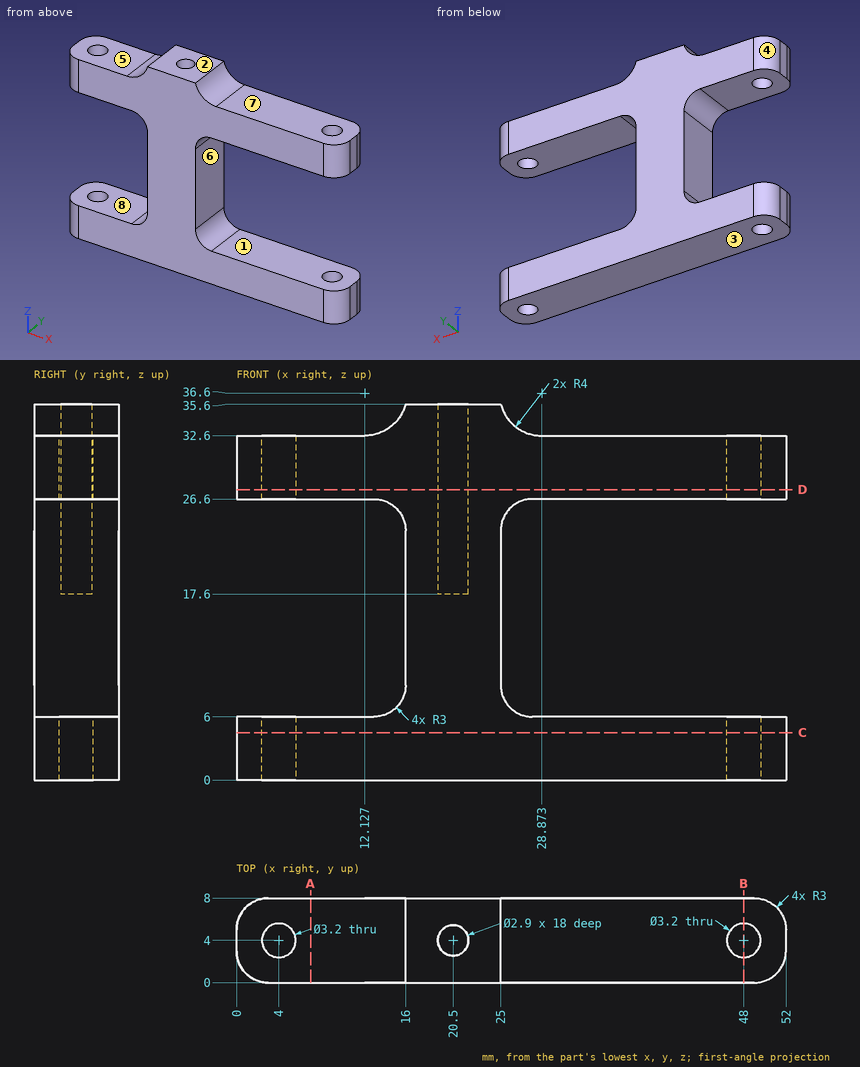
Study the drawing (mm; zero at the part's minimum x, y, z) and answer. A direction names the side the tool comes from. Round coordinates to 2 decimals unless told otherwise and drop trailing zeros. Write each loop counter-clockwise with the first axis right and the second up, starting at its lowest first coordinate (ties: lowest second). Pieces come first, ordered by that corner, then holes.
Q1. The mould has two halves that part along Z. Classify the marked faces 1, 2, 3 and 4: released by +Z, released by -Z, zero draft, split by the parting line, or undercut.
Values:
face 1: undercut
face 2: released by +Z
face 3: released by -Z
face 4: zero draft
Q2. Find section A-A on x = 7. Determine the outline of the cut face in (y, z), and give its area (3 significant figures).
Values:
outline: (0, 0) - (8, 0) - (8, 6) - (0, 6) - close; (0, 26.6) - (8, 26.6) - (8, 32.6) - (0, 32.6) - close
area: 96.0 mm2
Q3. Straight lines are drawn through the part: line 1 (Z direction, x = 33, y = 1.5); line 2 (Y direction, x = 48, z = 1.65); line 3 (X direction, y = 2.75, z = 31) (1 decimal). For each, find the intervals that lie inside material, in ascending order.
Values:
line 1: z = 0 to 6, 26.6 to 32.6
line 2: y = 0 to 2.4, 5.6 to 8
line 3: x = 0 to 3, 5 to 19.8, 21.2 to 47, 49 to 52
Q4. Find section B-B on x = 48. Determine the outline of the cut face in (y, z), and give its area (3 significant figures).
Values:
outline: (0, 0) - (2.4, 0) - (2.4, 6) - (0, 6) - close; (0, 26.6) - (2.4, 26.6) - (2.4, 32.6) - (0, 32.6) - close; (5.6, 0) - (8, 0) - (8, 6) - (5.6, 6) - close; (5.6, 26.6) - (8, 26.6) - (8, 32.6) - (5.6, 32.6) - close
area: 57.6 mm2
Q5. Find section C-C on z = 4.5. Determine the outline of the cut face in (x, y), and give its area (3 significant figures).
Values:
outline: (0, 3) arc R3 ccw to (3, 0) - (49, 0) arc R3 ccw to (52, 3) - (52, 5) arc R3 ccw to (49, 8) - (3, 8) arc R3 ccw to (0, 5) - close; hole circle Ø3.2 at (4, 4); hole circle Ø3.2 at (48, 4)
area: 392 mm2
Q6. Find section D-D on z = 27.5. Determine the outline of the cut face in (x, y), and give its area (3 significant figures).
Values:
outline: (0, 3) arc R3 ccw to (3, 0) - (49, 0) arc R3 ccw to (52, 3) - (52, 5) arc R3 ccw to (49, 8) - (3, 8) arc R3 ccw to (0, 5) - close; hole circle Ø3.2 at (4, 4); hole circle Ø2.9 at (20.5, 4); hole circle Ø3.2 at (48, 4)
area: 386 mm2
Q7. A tool of negligible diameter and unlimited length cuts with its end or side. For the marked faces 5, 6, 7 and 8, from which of +Z, -Z, +X, -X, +Y, -Y can it reach the whole face along a straight path? Write none if from no direction.
Values:
face 5: +Z, -X, +Y, -Y
face 6: +X, +Y, -Y
face 7: +Z, +X, +Y, -Y
face 8: -X, +Y, -Y
Q8. Flat-ended cylindrical pins translate along their axes: P1, Ø1.9, axis at x = 48, y = 4, coming from the -Z side (3 decimals); P2, Ø2.5, axis at x = 8.5, y = 2.5, coming from the +Z side; P3, Ø0.9, axis at x = 21, y = 4.5, coming from the +Z side; P4, Ø1.5, axis at y = 2, z = 9, coming from the +X side. Find the tip coordinate at first contact, or state that the pin passes through.
Values:
P1: passes through
P2: stops at z = 32.6
P3: stops at z = 17.6
P4: stops at x = 25.1
